Autodesk Inventor part; units mm, degrees
ref_plane "YZ Plane" through (0, 0, 0) normal (1, 0, 0) x (0, 1, 0)
ref_plane "XZ Plane" through (0, 0, 0) normal (0, 1, 0) x (-1, 0, 0)
ref_plane "XY Plane" through (0, 0, 0) normal (0, 0, 1) x (1, 0, 0)
sketch "Sketch1" plane through (0, 0, 0) normal (0, 1, 0) x (-1, 0, 0)
  line L0 (25, 25) -> (-25, 25)
  line L1 (-25, 25) -> (-25, -25)
  line L2 (-25, -25) -> (25, -25)
  line L3 (25, -25) -> (25, 25)
  line L4 (25, 25) -> (-25, -25) construction
  line L5 (-25, 25) -> (25, -25) construction
  line L6 (24, 24) -> (-24, 24)
  line L7 (-24, 24) -> (-24, -24)
  line L8 (-24, -24) -> (24, -24)
  line L9 (24, -24) -> (24, 24)
  line L10 (24, 24) -> (-24, -24) construction
  line L11 (-24, 24) -> (24, -24) construction
  point P0 (0, 0)
  dimension "d0" = 50
  dimension "d2" = 48
extrude "Extrusion1" add sketch "Sketch1" along normal blind 400
sketch "Sketch3" plane through (25, 0, -25) normal (0, 0, -1) x (-1, 0, 0)
  line L0 (50, 0) -> (50, 400)
  line L1 (0, 0) -> (0, 400)
  line L2 (50, 0) -> (50, 400)
  line L3 (0, 400) -> (50, 400)
  line L4 (50, 400) -> (50, 370)
  line L5 (50, 370) -> (0, 370)
  line L6 (0, 370) -> (0, 400)
  line L7 (0, 400) -> (50, 370) construction
  line L8 (25, 385) -> (40, 385) construction
  line L9 (25, 385) -> (10, 385) construction
  line L10 (0, 30) -> (50, 30)
  line L11 (50, 30) -> (50, 0)
  line L12 (50, 0) -> (0, 0)
  line L13 (0, 0) -> (0, 30)
  line L14 (0, 30) -> (50, 0) construction
  circle A0 centre (40, 15) radius 2
  line L15 (25, 15) -> (40, 15) construction
  line L16 (25, 15) -> (10, 15) construction
  circle A1 centre (10, 15) radius 2
  line L17 (25, 385) -> (25, 345) construction
  circle A2 centre (25, 345) radius 6
  line L18 (25, 345) -> (36.3137, 333.6863) construction
  line L19 (0, 0) -> (16, 0) construction
  line L20 (25, 345) -> (13.6863, 356.3137) construction
  circle A3 centre (36.3137, 333.6863) radius 2.5
  circle A4 centre (13.6863, 356.3137) radius 2.5
  circle A5 centre (36.3137, 356.3137) radius 2.5
  circle A6 centre (13.6863, 333.6863) radius 2.5
  dimension "d28" = 30
  dimension "d30" = 15
  dimension "d31" = 15
  dimension "d33" = 30
  dimension "d34" = 4
  dimension "d35" = 15
  dimension "d36" = 15
  dimension "d37" = 4
  dimension "d38" = 40
  dimension "d61" = 12
  dimension "d64" = 16
  dimension "d65" = 5
extrude "Extrusion3" cut sketch "Sketch3" against normal blind 50 contours A0 | A1 | A2 | A3 | A4 | A5 | A6
sketch "Sketch5" plane through (25, 0, 25) normal (1, 0, 0) x (0, 0, -1)
  line L0 (0, 400) -> (50, 400)
  line L1 (50, 400) -> (50, 370)
  line L2 (50, 370) -> (0, 370)
  line L3 (0, 370) -> (0, 400)
  line L4 (0, 400) -> (50, 370) construction
  circle A0 centre (40, 385) radius 2
  line L5 (25, 385) -> (40, 385) construction
  line L6 (25, 385) -> (10, 385) construction
  circle A1 centre (10, 385) radius 2
  point P0 (25, 0)
  dimension "d40" = 30
  dimension "d41" = 4
  dimension "d42" = 15
  dimension "d43" = 15
  dimension "d44" = 4
extrude "Extrusion5" cut sketch "Sketch5" against normal blind 50 contours A0 | A1
properties part number "End-Link" material "Aluminum 6061"
Work out the finished part from the listing and answer in its coordinate system (mm). A direction names the side the tool comes from. Coordinates: 2 decimals unless noted, no trailing zeros. Write each loop counter-clockwise with the first axis right and the second up, starting at its lowest first coordinate (ties: lowest second). Pieces come first, ordered by that corner, then holes.
1. The part is cut by section A-A, the plane z = 1. Write down the section's boundary in (x, y).
Results list:
outline: (-25, 0) - (-24, 0) - (-24, 400) - (-25, 400) - close; (24, 0) - (25, 0) - (25, 400) - (24, 400) - close
2. For a pull along Y with two mould halves and no side action, classify faces 3 (the flat face through (0, 197, 25)), 4 (the flat face through (24.2, 0, 11.2)), 5 (the cylindrical face through (0.78, 350.95, 24.49)), 6 (the cylindrical face through (0.78, 350.95, -24.51)) as +Y half, -Y half, draft (parallel to the pull), parting line (faces both ways), or undercut.
Results list:
face 3: draft
face 4: -Y half
face 5: undercut
face 6: undercut
3. The part is cut by section B-B, the plane x = 0. Write down the section's boundary in (y, z), and give its area (3 significant figures).
Results list:
outline: (0, -25) - (339, -25) - (339, -24) - (0, -24) - close; (0, 24) - (339, 24) - (339, 25) - (0, 25) - close; (351, -25) - (400, -25) - (400, -24) - (351, -24) - close; (351, 24) - (400, 24) - (400, 25) - (351, 25) - close
area: 776 mm2
4. Consider line 1 along X through (y, z) = (256, -5); line 2 along Y through (x, z) = (-24.4, -15). Determine where each line is inside the solid, lowest interval first.
Results list:
line 1: x = -25 to -24, 24 to 25
line 2: y = 0 to 383, 387 to 400
5. For faces 1 (the flat face through (0, 197, 24)), 2 (the flat face through (25, 197, 0)), determine the directions among +Z, -Z, +X, -X, +Y, -Y from which every point of the face is accessible in a straight line to the end or side of a thin tool.
Results list:
face 1: +Y, -Y
face 2: +Z, -Z, +X, +Y, -Y
6. The part is cut by section C-C, the plane y = 259.5. Write down the section's boundary in (x, z), and give its area (3 significant figures).
Results list:
outline: (-25, -25) - (25, -25) - (25, 25) - (-25, 25) - close; hole (-24, -24) - (24, -24) - (24, 24) - (-24, 24) - close
area: 196 mm2
